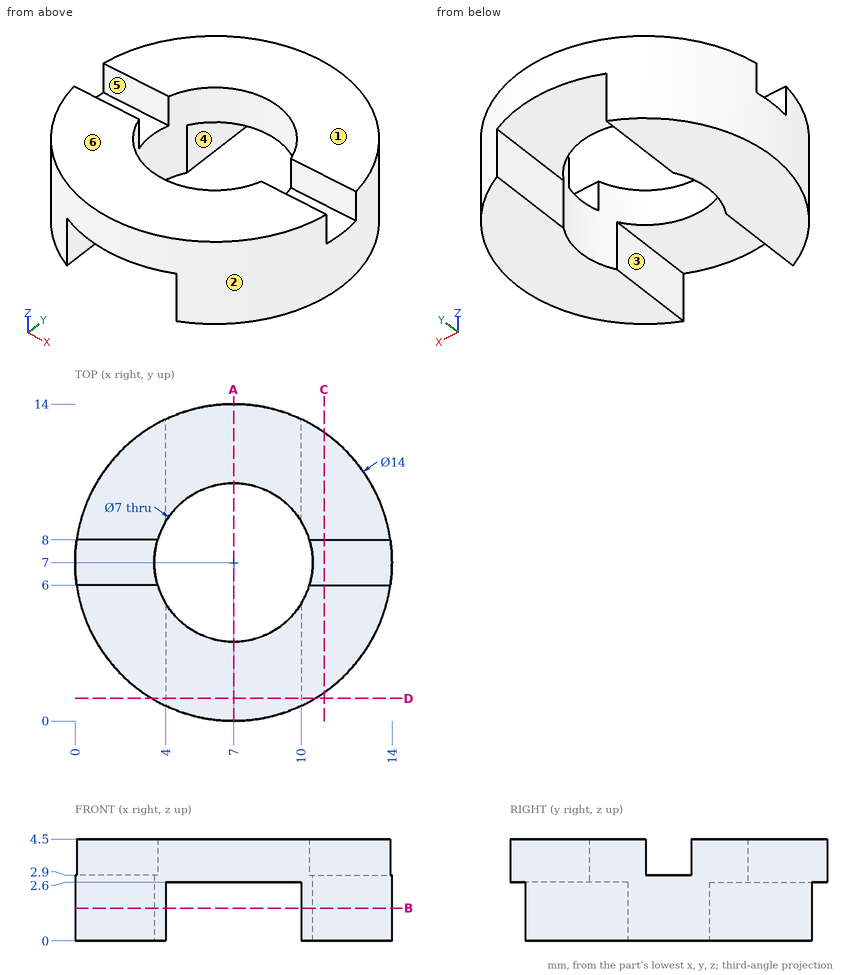
Check sheet for the drawn part. Datum: minimum x, y, z corner. Units: mm. A direction names the side the tool comes from. Coordinates: 2 decimals unless noted, no trailing zeros. Loops run counter-clockwise (first coordinate to the right, second up) from the corner with the lowest first, then second, coordinate; pieces in that order, holes last. Notation, with made-up numbers: (87, -2) - (127, -2) arc R16 ccw to (127, 18) - close; hole circle Ø5 at (-6.5, 56). An arc over 180 degrees is marked (long way). Put each result on its own line as item: value.
Item 1: Section check C-C (x = 11). Enter the section's corners in (y, z).
Conclusion:
outline: (1.26, 0) - (12.74, 0) - (12.74, 4.5) - (8, 4.5) - (8, 2.9) - (6, 2.9) - (6, 4.5) - (1.26, 4.5) - close
Item 2: Section check B-B (z = 1.45). Enter the section's corners in (x, y), then the cut area to 3 significant figures.
Conclusion:
outline: (4, 0.68) - (4, 5.2) arc R3.5 cw to (4, 8.8) - (4, 13.32) arc R7 ccw to start; (10, 0.68) arc R7 ccw to (10, 13.32) - (10, 8.8) arc R3.5 cw to (10, 5.2) - close
area: 70.1 mm2
Item 3: Section check D-D (y = 1). Enter the section's corners in (x, z).
Conclusion:
outline: (3.39, 0) - (4, 0) - (4, 2.6) - (10, 2.6) - (10, 0) - (10.61, 0) - (10.61, 4.5) - (3.39, 4.5) - close
Item 4: Scan lines: line 1 along X through (y, z) = (7, 2.55); line 2 along Y through (x, z) = (6, 2.65). Record each from-to range of solid material in increasing order.
Conclusion:
line 1: x = 0 to 3.5, 10.5 to 14
line 2: y = 0.07 to 3.65, 10.35 to 13.93
Item 5: Gauge pin test, flat ends, axial feed: pin 1 Ø1.3 at (y, z) = (10.5, 1) entering from -X; pin 2 Ø2 at (y, z) = (3, 1) entering from +X; pin 3 Ø1.8 at (x, z) = (2, 3.5) entering from +Y. Record the tip position at first contact, or that the pin passes through.
Conclusion:
pin 1: stops at x = 0.61
pin 2: stops at x = 13.32
pin 3: stops at y = 12.67
Item 6: Set-up check for the marked faces 4, 5 and 6: record each of +Z, -Z, +X, -X, +Y, -Y from which the full face is reachable in a straight line by a thin tool's end or side.
Conclusion:
face 4: -Z, +Y, -Y
face 5: +Z, +X, -X
face 6: +Z, +X, -X, +Y, -Y
Item 7: Section check A-A (x = 7). Enter the section's corners in (y, z).
Conclusion:
outline: (0, 2.6) - (3.5, 2.6) - (3.5, 4.5) - (0, 4.5) - close; (10.5, 2.6) - (14, 2.6) - (14, 4.5) - (10.5, 4.5) - close
Item 8: Draft check along X on the marked faces 1, 2 and 3. Enter one of: pulls with the +X half, pulls with the -X half, needs draft (parallel to the pull), parting line crosses it, or undercut.
Conclusion:
face 1: needs draft
face 2: parting line crosses it
face 3: undercut
